Input: part model. Units: mm. Frame: model coordinates. A direction names the side the tool comes from. Round coordinates to 2 decimals unless told otherwise and drop trailing zeros. Loops run counter-clockwise (first coordinate to the right, second up) from the corner with the lowest first, then second, coordinate; pieces in that order, holes last.
(1) First-contact query: pin 1 Ø5 at (x, y) = (7.5, 18) entering from -Z; pin 2 Ø8.5 at (x, z) = (0, 0) entering from -Y; pin 3 Ø1.5 at (y, z) = (34, 7.5) entering from -X. Flat tips, straight axial feed; report the tip coordinate or a pass-through.
(2) Cut plane A-A, the plane x = 0. Output: boundary loops of the cut face in (y, z), and give its area (3 significant figures).
(3) Access query for faces 1 (the face through (0, 2.286, 0)), 2 (the face through (4, 0, 4)). Directions: +Z, -Z, +X, -X, +Y, -Y. A direction counts if a zero-diameter tool reaches every point of the face in a straight line with its end or side. Return the directions, or none.
(4) Cut plane C-C, the plane y = 6. Output: boundary loops of the cut face in (x, z), and give its area (3 significant figures).
(5) Draft query along X for faces 3 (the face through (-2.842, 28.964, -9.025)), 4 (the face through (-1.438, 1.002, -4.567)), 5 (the face through (0, 57.15, 0)). Return one class per face: released by +X, released by -X, zero draft, split by the parting line, or undercut.
(6) Cut plane B-B, the plane z = 0. Output: boundary loops of the cut face in (x, y), and give its area (3 significant figures).
(7) Line query: line 1 (X direction, y = 1, z = 0); line 2 (Y direction, x = -1.75, z = 2); line 3 (Z direction, x = 0.25, y = 16). Output: solid intervals per line, ascending.
from build123d import *


with BuildPart() as part:
    # Sketch1 → Revolve1 (revolve)
    with BuildSketch(Plane.XY, mode=Mode.PRIVATE) as revolve1_sk:
        Polygon((9.4615, 0.762), (9.4615, 56.388), (8.6995, 57.15), (0, 57.15), (0, 2.286), (4.5339, 2.286), (4.7879, 2.032), (4.7879, 0), (8.6995, 0), align=None)
    revolve(revolve1_sk.sketch.rotate(Axis((0, 0, 0), (0, 1, 0)), 90), axis=Axis((0, 0, 0), (0, 1, 0)))  # turned: the seam where the file's is


solid = part.part
Reported:
1. pin 1: stops at z = -8.03
1. pin 2: stops at y = 2.29
1. pin 3: stops at x = -6.63
2. outline: (0, -8.7) - (0.76, -9.46) - (56.39, -9.46) - (57.15, -8.7) - (57.15, 8.7) - (56.39, 9.46) - (0.76, 9.46) - (0, 8.7) - (0, 4.79) - (2.03, 4.79) - (2.29, 4.53) - (2.29, -4.53) - (2.03, -4.79) - (0, -4.79) - close
2. area: 1,060 mm2
3. face 1: -Y
3. face 2: +Z, -Z, +X, -X, -Y
4. outline: circle Ø18.92 at (0, 0)
4. area: 281 mm2
5. face 3: split by the parting line
5. face 4: undercut
5. face 5: zero draft
6. outline: (-9.46, 0.76) - (-8.7, 0) - (-4.79, 0) - (-4.79, 2.03) - (-4.53, 2.29) - (4.53, 2.29) - (4.79, 2.03) - (4.79, 0) - (8.7, 0) - (9.46, 0.76) - (9.46, 56.39) - (8.7, 57.15) - (-8.7, 57.15) - (-9.46, 56.39) - close
6. area: 1,060 mm2
7. line 1: x = -9.46 to -4.79, 4.79 to 9.46
7. line 2: y = 2.29 to 57.15
7. line 3: z = -9.46 to 9.46
